from build123d import *

# Parameters (mm, degrees)
F0_W     = 12.7
F0_H     = 254
F1_DEPTH = 444.5
F2_W     = 101.6
F2_H     = 76.2
F3_DEPTH = 12.7
F4_W     = 25.4
F4_H     = 19.05
F4_W_2   = 12.7
F4_H_2   = 76.2
F5_DEPTH = 69.85
F6_W     = 12.7
F6_H     = 76.2
F7_DEPTH = 539.75
F8_W     = 539.75
F8_H     = 25.4
F9_DEPTH = 19.05


with BuildPart() as f1:
    # F0 (on Top) → F1 (new body)
    with BuildSketch(Plane.XY):
        with Locations((6.35, -139.7)):
            Rectangle(F0_W, F0_H)
        Polygon((12.7, -266.7), (0, -266.7), (0, -279.4), (565.15, -279.4), (565.15, -266.7), (552.45, -266.7), align=None)
        with Locations((558.8, -139.7)):
            Rectangle(F0_W, F0_H)
    extrude(amount=F1_DEPTH)

    # F2 (on face) → F3 (cut, through all)
    with BuildSketch(Plane(origin=(0, 0, 0), x_dir=(0, -1, 0), z_dir=(-1, 0, 0))):
        with Locations((50.8, 38.1)):
            Rectangle(F2_W, F2_H)
    extrude(amount=-F3_DEPTH, mode=Mode.SUBTRACT)

    # F4 (on face) → F5 (join)
    with BuildSketch(Plane(origin=(0, 0, 0), x_dir=(0, -1, 0), z_dir=(-1, 0, 0))):
        Polygon((101.6, 0), (114.3, 0), (114.3, 88.9), (12.7, 88.9), (12.7, 76.2), (38.1, 76.2), (88.9, 76.2), (101.6, 76.2), align=None)
        with Locations((25.4, 66.675)):
            Rectangle(F4_W, F4_H)
        with Locations((95.25, 38.1)):
            Rectangle(F4_W_2, F4_H_2)
    extrude(amount=F5_DEPTH)

    # F6 (on face) → F7 (join, through all)
    with BuildSketch(Plane(origin=(552.45, 0, 0), x_dir=(0, -1, 0), z_dir=(-1, 0, 0))):
        with Locations((19.05, 406.4)):
            Rectangle(F6_W, F6_H)
    extrude(amount=F7_DEPTH)

    # F8 (on face) → F9 (join)
    with BuildSketch(Plane.XY.offset(444.5)):
        with Locations((282.575, -38.1)):
            Rectangle(F8_W, F8_H)
        Polygon((565.15, -12.7), (0, -12.7), (0, -50.8), (12.7, -50.8), (12.7, -25.4), (552.45, -25.4), (552.45, -50.8), (565.15, -50.8), align=None)
    extrude(amount=F9_DEPTH)


solid = f1.part
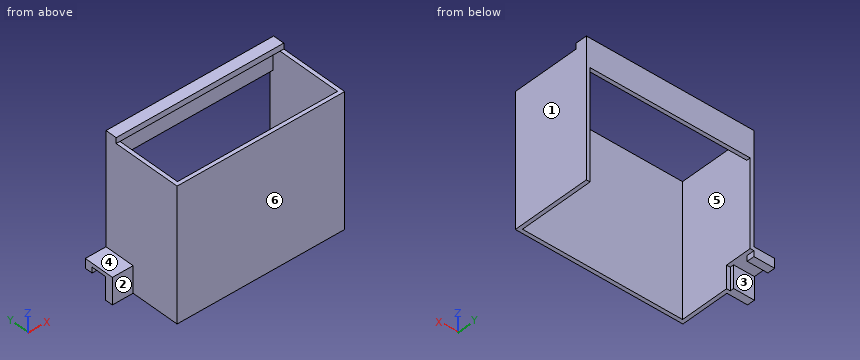
For this review, take the finished solid that the model builds, in its own axes (mm). Face numbers are marked on the shaded views. A direction names the side the tool comes from. Round coordinates to 2 decimals unless told otherwise and drop trailing zeros. Loops run counter-clockwise (first coordinate to the right, second up) from the corner with the lowest first, then second, coordinate; pieces in that order, holes last. Notation, with made-up numbers: (-25, -35) - (-6, -35) arc R27 ccw to (-6, -9) - close; hole circle Ø7 at (41, 70.25). An arc over 180 degrees is marked (long way). Put each result on its own line as item: value. Start each with the question number.
1. Insertion check: P1, Ø4, axis at y = -133, z = 216, coming from the -X side; P2, Ø10, axis at x = 351, y = -18, coming from the -Z side; P3, Ø21, axis at x = -38.5, y = -63.5, coming from the +Z side. Each pin has a flat end and moves straight along its axis. Give the tip position at first contact, or say it passes through.
2. Mouldability with a two-part tool opening along Y and no side actions: class the marked faces 4, 5 and 6 as +Y half, -Y half, draft (parallel to the pull), parting line (faces both ways), or undercut.
3. Consider section A-A on x = 118.5. State the section outline as (y, z) points, plus the area to 3 significant figures.
4. For probe 1 along X at (y, z) = (-142, 132); probe 2 along Y at (x, z) = (241.5, 391); probe 3 along X at (y, z) = (-89, 81.5), list the stretches that pass through material, from the lowest coordinate up. Write a range as [from, to].
5. Consider section D-D on y = -58.5. State the section outline as (x, z) points, plus the area to 3 significant figures.
6. Consider section B-B on y = -183. State the section outline as (x, z) points.
7. Consider section C-C on z = 107. State the section outline as (x, y) points.
8. For the marked faces 1, 2 and 3, list the 3-axis set-ups (+Z, -Z, +X, -X, +Y, -Y) from which the entire face can be reached by the end or side of a thin tool; tool diameter is ignored.
Result sheet:
1. P1: x = 0
1. P2: z = 368.3
1. P3: z = 88.9
2. face 4: draft
2. face 5: undercut
2. face 6: -Y half
3. outline: (-279.4, 0) - (-266.7, 0) - (-266.7, 444.5) - (-279.4, 444.5) - close; (-50.8, 444.5) - (-25.4, 444.5) - (-25.4, 368.3) - (-12.7, 368.3) - (-12.7, 463.55) - (-50.8, 463.55) - close
3. area: 7,340 mm^2
4. probe 1: [0, 12.7], [552.45, 565.15]
4. probe 2: [-279.4, -266.7], [-25.4, -12.7]
4. probe 3: [-69.85, 12.7], [552.45, 565.15]
5. outline: (-69.85, 76.2) - (12.7, 76.2) - (12.7, 444.5) - (0, 444.5) - (0, 88.9) - (-69.85, 88.9) - close; (552.45, 0) - (565.15, 0) - (565.15, 444.5) - (552.45, 444.5) - close
5. area: 11,200 mm^2
6. outline: (0, 0) - (12.7, 0) - (12.7, 444.5) - (0, 444.5) - close; (552.45, 0) - (565.15, 0) - (565.15, 444.5) - (552.45, 444.5) - close
7. outline: (0, -279.4) - (565.15, -279.4) - (565.15, -12.7) - (552.45, -12.7) - (552.45, -266.7) - (12.7, -266.7) - (12.7, -12.7) - (0, -12.7) - close
8. face 1: +Z, -Z, +X, +Y, -Y
8. face 2: +Z, -Z, -X, -Y
8. face 3: -Z, -X
